```python
from build123d import *

# Parameters (mm, degrees)
SKETCH4_R           = 62.5
SKETCH4_R_2         = 4
BOSS_EXTRUDE2_DEPTH = 15
CUT_EXTRUDE1_DEPTH  = 50


with BuildPart() as part:
    # Sketch3 → Revolve1 (revolve)
    with BuildSketch(Plane.XY):
        Polygon((0, 15), (62.5, 15), (40, 65), (15, 65), (15, 80), (0, 80), (0, 65), align=None)
    revolve(axis=Axis((0, 65, 0), (0, -1, 0)))

    # Sketch4 → Boss-Extrude2 (add)
    with BuildSketch(Plane.XZ.offset(-15)):
        Circle(SKETCH4_R)
        with Locations((52.5, 0)):
            Circle(SKETCH4_R_2, mode=Mode.SUBTRACT)
        with Locations((0, -52.5)):
            Circle(SKETCH4_R_2, mode=Mode.SUBTRACT)
        with Locations((-52.5, 0)):
            Circle(SKETCH4_R_2, mode=Mode.SUBTRACT)
        with Locations((0, 52.5)):
            Circle(SKETCH4_R_2, mode=Mode.SUBTRACT)
    extrude(amount=BOSS_EXTRUDE2_DEPTH)

    # Sketch4_5 → Cut-Extrude1 (cut)
    with BuildSketch(Plane.XZ.offset(-15)):
        with BuildLine():
            Line((7.480842881, -62.050680817), (7.480842881, -51.964285714))
            ThreePointArc((7.480842881, -51.964285714), (0, -45), (-7.480842881, -51.964285714))
            Line((-7.480842881, -51.964285714), (-7.480842881, -62.050680817))
            ThreePointArc((-7.480842881, -62.050680817), (0, -62.5), (7.480842881, -62.050680817))
        make_face()
        with BuildLine():
            Line((51.964285714, -7.480842881), (62.050680817, -7.480842881))
            ThreePointArc((62.050680817, -7.480842881), (62.5, 0), (62.050680817, 7.480842881))
            Line((62.050680817, 7.480842881), (51.964285714, 7.480842881))
            ThreePointArc((51.964285714, 7.480842881), (45, 0), (51.964285714, -7.480842881))
        make_face()
        with BuildLine():
            ThreePointArc((-62.050680817, 7.480842881), (-62.5, 0), (-62.050680817, -7.480842881))
            Line((-62.050680817, -7.480842881), (-51.964285714, -7.480842881))
            ThreePointArc((-51.964285714, -7.480842881), (-45, 0), (-51.964285714, 7.480842881))
            Line((-51.964285714, 7.480842881), (-62.050680817, 7.480842881))
        make_face()
        with BuildLine():
            ThreePointArc((7.480842881, 62.050680817), (0, 62.5), (-7.480842881, 62.050680817))
            Line((-7.480842881, 62.050680817), (-7.480842881, 51.964285714))
            ThreePointArc((-7.480842881, 51.964285714), (0, 45), (7.480842881, 51.964285714))
            Line((7.480842881, 51.964285714), (7.480842881, 62.050680817))
        make_face()
    extrude(amount=-CUT_EXTRUDE1_DEPTH, mode=Mode.SUBTRACT)


solid = part.part
```
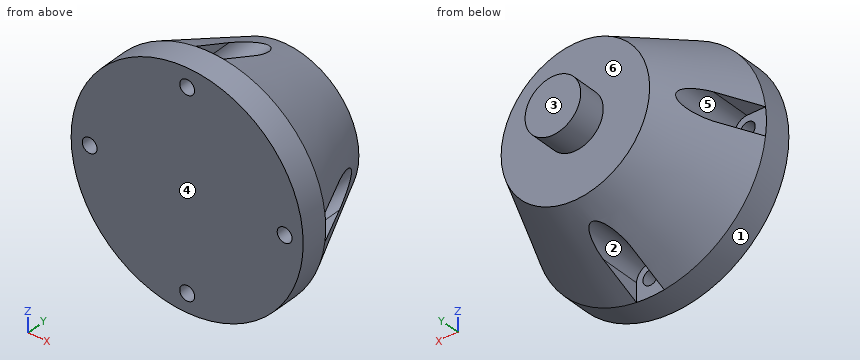
The listing builds one solid part. Answer for the finished solid, in the listing's coordinates (mm). Face numbers are marked on the shaded views. A direction names the side the tool comes from. Give positions to 0.01 mm unless a question says otherwise; leave off trailing zeros. Order: outer loops, then holes, each group sorted by start corner. A loop starts at its lowest first (then second) coordinate and runs counter-clockwise, first axis right, second up. Notation, with made-up numbers: (47.5, 66.25) -> (96.5, 66.25) arc R18 ccw to (96.5, 100.25) -> close; hole circle Ø4 at (72, 55). An arc over 180 degrees is marked (long way). Answer as a JSON object with one key per item and string values. Group by question number.
Item 1: Determine the mould class of the marked faces 1, 2 and 3 for opening direction X: pulls with the +X half, pulls with the -X half, needs draft (parallel to the pull), parting line crosses it, or undercut.
Item 2: The part is cut by section A-A on x = 0. Write down the section's boundary in (y, z).
Item 3: Consider L1, parallel to Z at x = 0, y = 10; L2, parallel to Y at x = 4.5, z = -57; L3, parallel to Y at x = 0, z = -19. Determine where each line is inside the solid, lowest interval first. Write a range as from..to.
Item 4: Flat-ended cylindrical pins translate along their axes: pin 1 (11 mm diameter, centred on x = -56, y = 22.5, fed in from -Z); pin 2 (7 mm diameter, centred on x = 0, z = -52.5, fed in from -Y); pin 3 (4.5 mm diameter, centred on x = 0.5, z = 56.5, fed in from +Y); pin 4 (1 mm diameter, centred on y = 34, z = -4, fed in from -X). Find the tip coordinate at first contact, or state that the pin passes through.
Item 5: A tool of negligible diameter and unlimited length cuts with its end or side. For the marked faces 4, 5 and 6, from which of +Z, -Z, +X, -X, +Y, -Y can it reach the whole face along a straight path? Write none if from no direction.
Item 6: The part is cut by section B-B on z = 0. Write down the section's boundary in (x, y), and give its area (3 significant figures).
Item 7: The part is cut by section D-D on y = 21.5. Write down the section's boundary in (x, z) (3 decimals).
Item 8: The part is cut by section C-C on y = 11.5. Write down the section's boundary in (x, z), and give its area (3 significant figures).
Result set:
{
 "1": {"face 1": "parting line crosses it", "face 2": "undercut", "face 3": "needs draft"},
 "2": {"outline": "(0, -62.5) -> (15, -62.5) -> (15, -56.5) -> (0, -56.5) -> close; (0, -48.5) -> (15, -48.5) -> (15, -45) -> (53.89, -45) -> (65, -40) -> (65, -15) -> (80, -15) -> (80, 15) -> (65, 15) -> (65, 40) -> (53.89, 45) -> (15, 45) -> (15, 48.5) -> (0, 48.5) -> close; (0, 56.5) -> (15, 56.5) -> (15, 62.5) -> (0, 62.5) -> close"},
 "3": {"L1": "-62.5..-56.5, -48.5..48.5, 56.5..62.5", "L2": "0..15", "L3": "0..65"},
 "4": {"pin 1": "z = -31.92", "pin 2": "through", "pin 3": "y = 15", "pin 4": "x = -46.5"},
 "5": {"face 4": "+Z, -Z, +X, -X, -Y", "face 5": "-X, +Y", "face 6": "+Y"},
 "6": {"outline": "(-62.5, 0) -> (-56.5, 0) -> (-56.5, 15) -> (-62.5, 15) -> close; (-48.5, 0) -> (48.5, 0) -> (48.5, 15) -> (45, 15) -> (45, 53.89) -> (40, 65) -> (15, 65) -> (15, 80) -> (-15, 80) -> (-15, 65) -> (-40, 65) -> (-45, 53.89) -> (-45, 15) -> (-48.5, 15) -> close; (56.5, 0) -> (62.5, 0) -> (62.5, 15) -> (56.5, 15) -> close", "area": "6,530 mm²"},
 "7": {"outline": "(-59.103, -7.481) arc R59.575 ccw to (-7.481, -59.103) -> (-7.481, -51.964) arc R7.5 cw to (7.481, -51.964) -> (7.481, -59.103) arc R59.575 ccw to (59.103, -7.481) -> (51.964, -7.481) arc R7.5 cw to (51.964, 7.481) -> (59.103, 7.481) arc R59.575 ccw to (7.481, 59.103) -> (7.481, 51.964) arc R7.5 cw to (-7.481, 51.964) -> (-7.481, 59.103) arc R59.575 ccw to (-59.103, 7.481) -> (-51.964, 7.481) arc R7.5 cw to (-51.964, -7.481) -> close"},
 "8": {"outline": "circle Ø125 at (0, 0); hole circle Ø8 at (-52.5, 0); hole circle Ø8 at (0, -52.5); hole circle Ø8 at (0, 52.5); hole circle Ø8 at (52.5, 0)", "area": "12,100 mm²"}
}
